Design review of the part built by this model. Coordinates are the model's own, in mm. Face numbers are marked on the shaded views. Coordinates: 2 decimals unless noted, no trailing zeros. Answer as CSV lines item,"result". Start each with the question number.
from build123d import *

# Parameters (mm, degrees)
F0_R            = 48.895
F1_DEPTH        = 6.35
F2_R            = 33.02
F3_DEPTH        = 3.175
F4_R            = 3.175
F5_DEPTH        = 6.351
F5_COPIES_COUNT = 3
F6_R            = 5.715
F7_DEPTH        = 3.175
F9_DEPTH        = 3.175


# Not quite as in the source:
# - a pattern or mirror of a feature is missing from the dataset's text; its kind, count and spacing are read off the source's solid


with BuildPart() as f1:
    # F0 (on Front) → F1 (new body)
    with BuildSketch(Plane.XZ):
        Circle(F0_R)
    extrude(amount=F1_DEPTH)

    # F2 (on face) → F3 (cut)
    with BuildSketch(Plane.XZ.offset(6.35)):
        Circle(F2_R)
    extrude(amount=-F3_DEPTH, mode=Mode.SUBTRACT)

    # F4 (on face) → F5 (cut, through all)
    with BuildSketch(Plane.XZ.offset(6.35)):
        with Locations((0, 41.275)):
            Circle(F4_R)
    f5 = extrude(amount=-F5_DEPTH, mode=Mode.SUBTRACT)

    # F5_copies: F5 ×3 about axis
    f5_copies_axis = Axis((0, 0, 0), (0, 1, 0))
    for i in range(1, F5_COPIES_COUNT):
        add(f5.rotate(f5_copies_axis, i * 360 / F5_COPIES_COUNT), mode=Mode.SUBTRACT)

    # F6 (on face) → F7 (cut)
    with BuildSketch(Plane.XZ.offset(6.35)):
        with Locations((0, 41.275)):
            Circle(F6_R)
        with Locations((35.7451985412, -20.6375)):
            Circle(F6_R)
        with Locations((-35.7451985412, -20.6375)):
            Circle(F6_R)
    extrude(amount=-F7_DEPTH, mode=Mode.SUBTRACT)

    # F8 (on face) → F9 (join)
    with BuildSketch(Plane.XZ.offset(3.175)):
        Polygon((-16.3922007191, 20.7727154884), (-28.2979620914, -11.5829327573), (-25.324323939, -11.5829327573), (-13.4185625667, 20.7727154884), align=None)
        Polygon((-16.905579319, -11.5829327573), (-6.9219360217, -11.5829327573), (4.9838253506, 20.7727154884), (-4.9998179467, 20.7727154884), align=None)
        Polygon((-12.4935675046, 20.7727154884), (-24.3993288769, -11.5829327573), (-17.8866158386, -11.5829327573), (-5.9808544663, 20.7727154884), align=None)
        with BuildLine():
            Line((5.8897674028, 20.7727154884), (2.173845637, 10.6741544806))
            Line((2.173845637, 10.6741544806), (12.9963092812, 10.6741544806))
            add(Edge.make_bspline(
                [(12.9963092812, 10.6741544806), (13.3555097893, 10.2684161805), (14.1043976934, 9.4225028304), (13.9491779559, 7.5181571268), (13.1134705599, 5.5267271878), (12.6059829763, 5.1538653523), (12.4124220311, 5.0116520418)],
                knots=[0, 0, 0, 0, 0.2524611124, 0.5263496824, 0.8193449335, 1, 1, 1, 1], degree=3))
            Line((12.4124220311, 5.0116520418), (0.2083620148, 5.0116520418))
            Line((0.2083620148, 5.0116520418), (-3.8432038956, -5.9990710312))
            Line((-3.8432038956, -5.9990710312), (5.090538634, -22.4072845116))
            Line((5.090538634, -22.4072845116), (19.059962988, -22.4072845116))
            Line((19.059962988, -22.4072845116), (22.3604289031, -11.5080620742))
            Line((22.3604289031, -11.5080620742), (14.3011480982, -11.5080620742))
            Line((14.3011480982, -11.5080620742), (10.3404486879, -4.2336190018))
            Line((10.3404486879, -4.2336190018), (19.6740036189, -4.2336190018))
            add(Edge.make_bspline(
                [(22.0640265758, 20.7727154884), (22.9280250832, 20.3392576633), (24.6989276358, 19.4508168126), (26.5202053139, 16.7535424772), (27.942801324, 12.3470202028), (27.4780031336, 7.7394644811), (26.2592507252, 2.6453616364), (23.4242960391, -1.5113689868), (20.9094052375, -3.3368697093), (19.6740036189, -4.2336190018)],
                knots=[0, 0, 0, 0, 0.1175129286, 0.2408614638, 0.3885970952, 0.5383784175, 0.6968239202, 0.8510693906, 1, 1, 1, 1], degree=3))
            Line((22.0640265758, 20.7727154884), (5.8897674028, 20.7727154884))
        make_face()
    extrude(amount=F9_DEPTH)

    # F10 (on Top) → F11 (revolve, cut)
    with BuildSketch(Plane.XY):
        Polygon((48.9125326276, -6.3948447905), (48.9125326276, 0), (48.2775326276, -6.3948447905), align=None)
    revolve(axis=Axis((0, -3.4167582635, 0), (0, -1, 0)), mode=Mode.SUBTRACT)


solid = f1.part
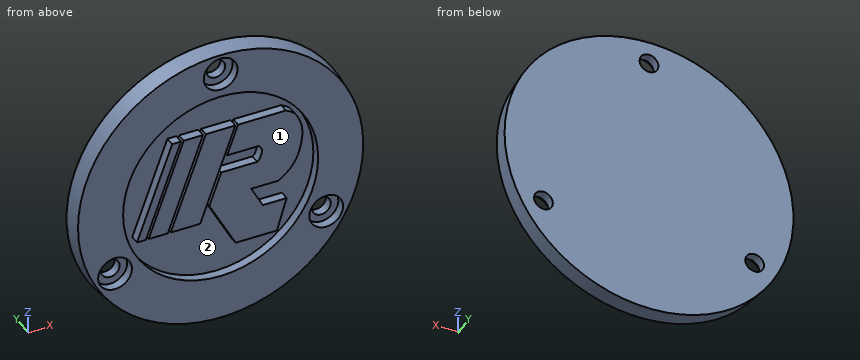
Item 1: For pin 1 (2.5 mm diameter, centred on x = -26.5, y = -4, fed in from -Z); pin 2 (10.5 mm diameter, centred on x = 0, z = 41.275, fed in from -Y) (3 decimals); pin 3 (2.5 mm diameter, centred on x = -21, y = -4.5, fed in from -Z), all flat-tipped, find the tip position at first contact; note any pin that passes through.
Item 2: Mouldability with a two-part tool opening along Z and no side actions: class the marked faces 1 and 2 as released by +Z, released by -Z, zero draft, split by the parting line, or undercut.
Item 3: Add section A-A (y = -4.5). Give the number of separate pieces and of enclosed holes in the cut face, plus the area to 3 significant figures.
Item 4: For line 1 along Z through (x, y) = (14.5, -3.5); line 2 along Z through (x, y) = (-36, -0.5); line 3 along X through (y, z) = (-5, -20.5), list the stretches that pass through material, from the lowest coordinate up. Write a range as from..to.
Response:
1,pin 1,"z = -41.44"
1,pin 2,"y = -3.175"
1,pin 3,"z = -44.28"
2,face 1,"zero draft"
2,face 2,"undercut"
3,separate pieces,"5"
3,enclosed holes,"4"
3,area,"5,130 mm²"
4,line 1,"-46.35..-29.67, -22.41..-11.51, -4.23..20.77, 29.67..46.35"
4,line 2,"-33.04..-23.8, -17.47..33.04"
4,line 3,"-43.86..-41.46, -30.03..-25.89, 4.05..19.64, 25.89..30.03, 41.46..43.86"
